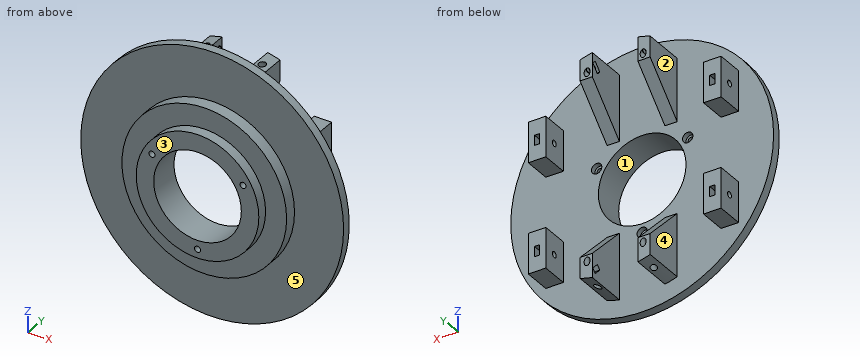
```python
from build123d import *

# Parameters (mm, degrees)
CROQUIS2_W                = 10
CROQUIS2_H                = 23
SALIENTE_EXTRUIR1_DEPTH   = 15.5
CROQUIS3_R                = 1.7
CORTAR_EXTRUIR1_DEPTH     = 15
CORTAR_EXTRUIR2_DEPTH     = 1.5
SIMETR_A2_COPY_1_SKETCH_W = 10
SIMETR_A2_COPY_1_SKETCH_H = 23
SIMETR_A2_COPY_1_DEPTH    = 15.5
SIMETR_A2_COPY_2_SKETCH_R = 1.7
SIMETR_A2_COPY_2_DEPTH    = 15
SIMETR_A2_COPY_3_DEPTH    = 1.5
CROQUIS5_R                = 1.7
CORTAR_EXTRUIR3_DEPTH     = 40.5
CROQUIS6_R                = 2.95
CORTAR_EXTRUIR4_DEPTH     = 3
MATRIZC1_COUNT            = 3
SALIENTE_EXTRUIR2_DEPTH   = 24
CORTAR_EXTRUIR5_DEPTH     = 10
CROQUIS9_R                = 1.7
CORTAR_EXTRUIR6_DEPTH     = 20
CORTAR_EXTRUIR7_DEPTH     = 3
SIMETR_A4_COPY_1_DEPTH    = 24
SIMETR_A4_COPY_2_DEPTH    = 10
SIMETR_A4_COPY_3_SKETCH_R = 1.7
SIMETR_A4_COPY_3_DEPTH    = 20
SIMETR_A4_COPY_4_DEPTH    = 3


with BuildPart() as part:
    # Croquis1 → Revolución1 (revolve)
    with BuildSketch(Plane.XY):
        Polygon((25, 0), (25, 18), (75, 18), (75, 13), (47, 13), (47, 6), (35, 6), (35, 0), align=None)
    revolve(axis=Axis((0, 49.685096011, 0), (0, -1, 0)))

    # Croquis2 → Saliente-Extruir1 (add)
    with BuildSketch(Plane(origin=(0, 18, 0), x_dir=(1, 0, 0), z_dir=(0, 1, 0))):
        with Locations((-50, -31.5)):
            Rectangle(CROQUIS2_W, CROQUIS2_H)
    saliente_extruir1 = extrude(amount=SALIENTE_EXTRUIR1_DEPTH)

    # Croquis3 → Cortar-Extruir1 (cut)
    with BuildSketch(Plane.ZY.offset(55)):
        with Locations((31.5, 26)):
            Circle(CROQUIS3_R)
    cortar_extruir1 = extrude(amount=-CORTAR_EXTRUIR1_DEPTH, mode=Mode.SUBTRACT)

    # Croquis4 → Cortar-Extruir2 (cut, symmetric)
    with BuildSketch(Plane.ZY.offset(50)):
        Polygon((28.598814897, 27.175), (28.598814897, 37.175), (34.401185103, 37.175), (34.401185103, 27.175), (34.401185103, 24.325), (31.5, 22.65), (28.598814897, 24.325), align=None)
    cortar_extruir2 = extrude(amount=CORTAR_EXTRUIR2_DEPTH, both=True, mode=Mode.SUBTRACT)

    # Simetría1: Saliente-Extruir1, Cortar-Extruir1, Cortar-Extruir2 across plane
    add(saliente_extruir1.mirror(Plane(origin=(0, 0, 0), x_dir=(0, 0, 1), z_dir=(1, 0, 0))))
    add(cortar_extruir1.mirror(Plane(origin=(0, 0, 0), x_dir=(0, 0, 1), z_dir=(1, 0, 0))), mode=Mode.SUBTRACT)
    add(cortar_extruir2.mirror(Plane(origin=(0, 0, 0), x_dir=(0, 0, 1), z_dir=(1, 0, 0))), mode=Mode.SUBTRACT)

    # Simetría2: Saliente-Extruir1, Cortar-Extruir1, Cortar-Extruir2 across plane
    add(saliente_extruir1.mirror(Plane.XY))
    add(cortar_extruir1.mirror(Plane.XY), mode=Mode.SUBTRACT)
    add(cortar_extruir2.mirror(Plane.XY), mode=Mode.SUBTRACT)

    # Simetría2 copy 1 sketch → Simetría2 copy 1 (add)
    with BuildSketch(Plane(origin=(0, 18, 0), x_dir=(-1, 0, 0), z_dir=(0, 1, 0))):
        with Locations((-50, -31.5)):
            Rectangle(SIMETR_A2_COPY_1_SKETCH_W, SIMETR_A2_COPY_1_SKETCH_H)
    extrude(amount=SIMETR_A2_COPY_1_DEPTH)

    # Simetría2 copy 2 sketch → Simetría2 copy 2 (cut)
    with BuildSketch(Plane(origin=(55, 0, 0), x_dir=(0, 0, -1), z_dir=(1, 0, 0))):
        with Locations((31.5, 26)):
            Circle(SIMETR_A2_COPY_2_SKETCH_R)
    extrude(amount=-SIMETR_A2_COPY_2_DEPTH, mode=Mode.SUBTRACT)

    # Simetría2 copy 3 sketch → Simetría2 copy 3 (cut, symmetric)
    with BuildSketch(Plane(origin=(50, 0, 0), x_dir=(0, 0, -1), z_dir=(1, 0, 0))):
        Polygon((28.598814897, 27.175), (28.598814897, 37.175), (34.401185103, 37.175), (34.401185103, 27.175), (34.401185103, 24.325), (31.5, 22.65), (28.598814897, 24.325), align=None)
    extrude(amount=SIMETR_A2_COPY_3_DEPTH, both=True, mode=Mode.SUBTRACT)

    # Croquis5 → Cortar-Extruir3 (cut)
    with BuildSketch(Plane(origin=(0, 18, 0), x_dir=(1, 0, 0), z_dir=(0, 1, 0))):
        with Locations((0, 30)):
            Circle(CROQUIS5_R)
    cortar_extruir3 = extrude(amount=-CORTAR_EXTRUIR3_DEPTH, mode=Mode.SUBTRACT)

    # Croquis6 → Cortar-Extruir4 (cut)
    with BuildSketch(Plane(origin=(0, 18, 0), x_dir=(1, 0, 0), z_dir=(0, 1, 0))):
        with Locations((0, 30)):
            Circle(CROQUIS6_R)
    cortar_extruir4 = extrude(amount=-CORTAR_EXTRUIR4_DEPTH, mode=Mode.SUBTRACT)

    # MatrizC1: Cortar-Extruir3, Cortar-Extruir4 ×3 about axis
    matrizc1_axis = Axis((0, 0, 0), (0, 1, 0))
    for i in range(1, MATRIZC1_COUNT):
        add(cortar_extruir3.rotate(matrizc1_axis, i * 360 / MATRIZC1_COUNT), mode=Mode.SUBTRACT)
        add(cortar_extruir4.rotate(matrizc1_axis, i * 360 / MATRIZC1_COUNT), mode=Mode.SUBTRACT)

    # Croquis7 → Saliente-Extruir2 (add)
    with BuildSketch(Plane(origin=(0, 18, 0), x_dir=(1, 0, 0), z_dir=(0, 1, 0))):
        with BuildLine():
            Line((13, 63.686733312), (13, 26))
            Line((13, 26), (20, 26))
            Line((20, 26), (20, 61.846584384))
            ThreePointArc((20, 61.846584384), (16.525632727, 62.864166764), (13, 63.686733312))
        make_face()
    saliente_extruir2 = extrude(amount=SALIENTE_EXTRUIR2_DEPTH)

    # Croquis8 → Cortar-Extruir5 (cut)
    with BuildSketch(Plane.ZY.offset(-13)):
        Polygon((-26, 18), (-71, 63), (-26, 63), align=None)
    cortar_extruir5 = extrude(amount=-CORTAR_EXTRUIR5_DEPTH, mode=Mode.SUBTRACT)

    # Croquis9 → Cortar-Extruir6 (cut)
    with BuildSketch(Plane(origin=(0, -4, -4), x_dir=(1, 0, 0), z_dir=(0, 0.707106781, 0.707106781))):
        with Locations((16, 67.553823869)):
            Circle(CROQUIS9_R)
    cortar_extruir6 = extrude(amount=-CORTAR_EXTRUIR6_DEPTH, mode=Mode.SUBTRACT)

    # Croquis10 → Cortar-Extruir7 (cut)
    with BuildSketch(Plane(origin=(0, -10.363961031, -10.363961031), x_dir=(1, 0, 0), z_dir=(0, 0.707106781, 0.707106781))):
        Polygon((17.675, 64.652638766), (19.35, 67.553823869), (17.675, 70.455008972), (14.325, 70.455008972), (7.675, 70.455008972), (7.675, 64.652638766), (14.325, 64.652638766), align=None)
    cortar_extruir7 = extrude(amount=CORTAR_EXTRUIR7_DEPTH, mode=Mode.SUBTRACT)

    # Simetría3: Saliente-Extruir2, Cortar-Extruir5, Cortar-Extruir6, Cortar-Extruir7 across plane
    add(saliente_extruir2.mirror(Plane(origin=(0, 0, 0), x_dir=(0, 0, 1), z_dir=(1, 0, 0))))
    add(cortar_extruir5.mirror(Plane(origin=(0, 0, 0), x_dir=(0, 0, 1), z_dir=(1, 0, 0))), mode=Mode.SUBTRACT)
    add(cortar_extruir6.mirror(Plane(origin=(0, 0, 0), x_dir=(0, 0, 1), z_dir=(1, 0, 0))), mode=Mode.SUBTRACT)
    add(cortar_extruir7.mirror(Plane(origin=(0, 0, 0), x_dir=(0, 0, 1), z_dir=(1, 0, 0))), mode=Mode.SUBTRACT)

    # Simetría4: Saliente-Extruir2, Cortar-Extruir5, Cortar-Extruir6, Cortar-Extruir7 across plane
    add(saliente_extruir2.mirror(Plane.XY))
    add(cortar_extruir5.mirror(Plane.XY), mode=Mode.SUBTRACT)
    add(cortar_extruir6.mirror(Plane.XY), mode=Mode.SUBTRACT)
    add(cortar_extruir7.mirror(Plane.XY), mode=Mode.SUBTRACT)

    # Simetría4 copy 1 sketch → Simetría4 copy 1 (add)
    with BuildSketch(Plane(origin=(0, 18, 0), x_dir=(-1, 0, 0), z_dir=(0, 1, 0))):
        with BuildLine():
            Line((13, 63.686733312), (13, 26))
            Line((13, 26), (20, 26))
            Line((20, 26), (20, 61.846584384))
            ThreePointArc((20, 61.846584384), (16.525632727, 62.864166764), (13, 63.686733312))
        make_face()
    extrude(amount=SIMETR_A4_COPY_1_DEPTH)

    # Simetría4 copy 2 sketch → Simetría4 copy 2 (cut)
    with BuildSketch(Plane(origin=(-13, 0, 0), x_dir=(0, 0, -1), z_dir=(1, 0, 0))):
        Polygon((-26, 18), (-71, 63), (-26, 63), align=None)
    extrude(amount=-SIMETR_A4_COPY_2_DEPTH, mode=Mode.SUBTRACT)

    # Simetría4 copy 3 sketch → Simetría4 copy 3 (cut)
    with BuildSketch(Plane(origin=(0, -4, 4), x_dir=(-1, 0, 0), z_dir=(0, 0.707106781, -0.707106781))):
        with Locations((16, 67.553823869)):
            Circle(SIMETR_A4_COPY_3_SKETCH_R)
    extrude(amount=-SIMETR_A4_COPY_3_DEPTH, mode=Mode.SUBTRACT)

    # Simetría4 copy 4 sketch → Simetría4 copy 4 (cut)
    with BuildSketch(Plane(origin=(0, -10.363961031, 10.363961031), x_dir=(-1, 0, 0), z_dir=(0, 0.707106781, -0.707106781))):
        Polygon((17.675, 64.652638766), (19.35, 67.553823869), (17.675, 70.455008972), (14.325, 70.455008972), (7.675, 70.455008972), (7.675, 64.652638766), (14.325, 64.652638766), align=None)
    extrude(amount=SIMETR_A4_COPY_4_DEPTH, mode=Mode.SUBTRACT)


solid = part.part
```
Could you check a few things on this model? Use its own coordinates, in mm. Face numbers are marked on the shaded views. A direction names the side the tool comes from. Coordinates: 2 decimals unless noted, no trailing zeros. Order: outer loops, then holes, each group sorted by start corner. A loop starts at its lowest first (then second) coordinate and runs counter-clockwise, first axis right, second up. Notation, with made-up numbers: M 84,44.5 L 106,44.5 A14 ccw 106,58.5 Z; hole C 59.25,51 d7. An arc over 180 degrees is marked long. Use a Markdown table: item, result. Add a question column.
Q1. I want a section at B-B on x = 42.5. List the corners of the cut face in (y, z) for me.
Q2. I want a section at A-A on z = -3. List the corners of the cut face in (x, y) for me.
Q3. We'd pull the mould along Z, two halves only. Please class the marked faces 1 and 2: pulls with the +Z half, pulls with the -Z half, needs draft (parallel to the pull), parting line crosses it, or undercut.
Q4. I'm going to push flat-ended pins straight in: pin 1 (5 mm diameter, centred on x = 49.5, y = 26, fed in from +Z); pin 2 (5.5 mm diameter, centred on y = 26, z = 31.5, fed in from -X); pin 3 (2 mm diameter, centred on y = 16.5, z = 54.5, fed in from -X). Where does each tip first touch, or does it pass through?
Q5. Which directions (+Z, -Z, +X, -X, +Y, -Y) give clear straight access to the entire face, cutting with the end or side of a thin tool? Please do the marked faces 3, 4 and 5.
Q6. If I drill on L1, parallel to X at y = 30.5, z = 41; L2, parallel to X at y = 37, z = -52; L3, parallel to Y at x = -26, z = -18, over which ranges is the centre line in solid material (lowest first)?
Checked values:
| question | item | result |
|---|---|---|
| 1 | outline | M 6,-20.07 L 13,-20.07 L 13,-61.8 L 18,-61.8 L 18,61.8 L 13,61.8 L 13,20.07 L 6,20.07 Z |
| 2 | outline | M -74.94,13 L -46.9,13 L -46.9,6 L -34.87,6 L -34.87,0 L -24.82,0 L -24.82,18 L -74.94,18 Z; M 24.82,0 L 34.87,0 L 34.87,6 L 46.9,6 L 46.9,13 L 74.94,13 L 74.94,18 L 24.82,18 Z |
| 3 | face 1 | undercut |
| 3 | face 2 | needs draft |
| 4 | pin 1 | z = 43 |
| 4 | pin 2 | x = -55 |
| 4 | pin 3 | x = -52.56 |
| 5 | face 3 | +Z, -Z, +X, -X, -Y |
| 5 | face 4 | +Z, -Z, +Y |
| 5 | face 5 | -Y |
| 6 | L1 | -55 to -45, -20 to -13, 13 to 20, 45 to 55 |
| 6 | L2 | -20 to -13, 13 to 20 |
| 6 | L3 | 0 to 18 |
